The listing builds one solid part. Answer for the finished solid, in the listing's coordinates (mm). Face numbers are marked on the shaded views. A direction names the side the tool comes from. Give positions to 0.01 mm unless a question says otherwise; leave off trailing zeros. Write each loop counter-clockwise with the first axis right and the second up, starting at its lowest first coordinate (ties: lowest second). Pieces come first, ordered by that corner, then holes. Notation, with made-up numbers: M -28,20 L -12,20 A28 cw -12,56 Z; hole C -16,-35.75 d4. An arc over 180 degrees is marked long. Return JSON: item names as keys, results as strings.
Autodesk Inventor part; units mm, degrees
ref_plane "YZ Plane" through (0, 0, 0) normal (1, 0, 0) x (0, 1, 0)
ref_plane "XZ Plane" through (0, 0, 0) normal (0, 1, 0) x (-1, 0, 0)
ref_plane "XY Plane" through (0, 0, 0) normal (0, 0, 1) x (1, 0, 0)
sketch "Sketch1" plane through (0, 0, 0) normal (0, 0, 1) x (1, 0, 0)
  line L0 (0, 0) -> (34, 0)
  line L1 (34, 0) -> (34, 20)
  line L2 (34, 20) -> (0, 20)
  line L3 (0, 20) -> (0, 0)
  circle A0 centre (29, 10) radius 2.5
  point P0 (34, 10)
  dimension "d0" = 34
  dimension "d1" = 20
  dimension "d2" = 5
  dimension "d3" = 5
extrude "Extrusion1" add sketch "Sketch1" along normal blind 5
sketch "Sketch2" plane through (0, 0, 0) normal (-1, 0, 0) x (0, 0, 1)
  line L0 (0, 0) -> (0, 20)
  line L1 (0, 20) -> (34, 20)
  line L2 (34, 20) -> (34, 0)
  line L3 (34, 0) -> (0, 0)
  line L4 (0, 0) -> (0, 20)
  circle A0 centre (29, 10) radius 2.5
  point P0 (5, 0)
  point P1 (34, 10)
  dimension "d6" = 34
  dimension "d7" = 5
  dimension "d8" = 5
extrude "Extrusion2" add sketch "Sketch2" against normal blind 5
sketch "Sketch3" plane through (0, 20, 0) normal (0, 1, 0) x (1, 0, 0)
  line L0 (34, -5) -> (5, -5)
  line L1 (5, -5) -> (5, -34)
  line L2 (5, -34) -> (5, -5)
  line L3 (5, -34) -> (34, -5)
  point P0 (0, 0)
extrude "Extrusion3" add sketch "Sketch3" against normal blind 2
sketch "Sketch4" plane through (0, 0, 0) normal (0, -1, 0) x (1, 0, 0)
  line L0 (34, 5) -> (5, 5)
  line L1 (34, 5) -> (5, 34)
  line L2 (5, 5) -> (5, 34)
  point P0 (0, 0)
extrude "Extrusion4" add sketch "Sketch4" against normal blind 2
sketch "Sketch5" plane through (0, 18, 0) normal (0, -1, 0) x (1, 0, 0)
  line L0 (5, 31.5) -> (5, 26.5)
  line L1 (26.5, 5) -> (31.5, 5)
  line L2 (5, 26.5) -> (5, 5)
  line L3 (5, 5) -> (26.5, 5)
  line L4 (5, 21) -> (21, 5)
  line L5 (29, 5) -> (29, 0)
  line L6 (34, 0) -> (0, 0)
  line L7 (5, 29) -> (0, 29)
  line L8 (5, 21) -> (18, 21)
  line L9 (21, 5) -> (21, 18)
  line L10 (5, 34) -> (34, 5)
  line L11 (18, 21) -> (21, 18)
  dimension "d15" = 8
  dimension "d16" = 8
extrude "Extrusion5" add sketch "Sketch5" along normal blind 16
properties part number "L Bracket Small"
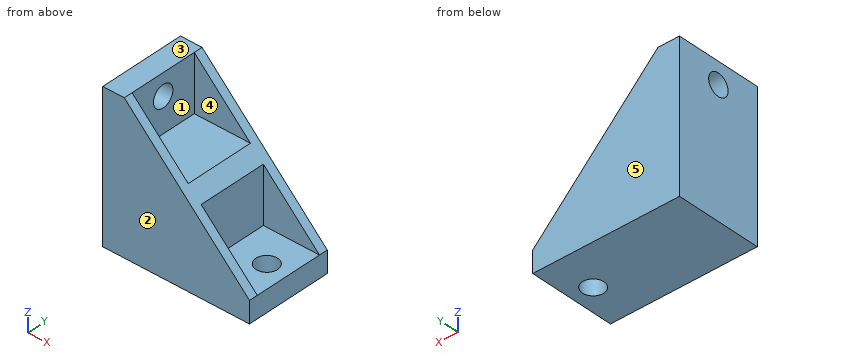
Item 1: A cutting plane is placed at D-D, the plane z = 22. Write down the section's boundary in (x, y).
Geometry results:
{"outline": "M 0,0 L 17,0 L 17,2 L 5,2 L 5,18 L 17,18 L 17,20 L 0,20 Z"}
Item 2: Which of the six approach directions +Z, -Z, +X, -X, +Y, -Y give full straight-line access (tool end or side, diameter ignored) to the marked faces 1 and 2?
Geometry results:
{"face 1": "+Z, +X", "face 2": "+Z, -Z, +X, -X, -Y"}
Item 3: A cutting plane is placed at C-C, the plane y = 10. Write down the section's boundary in (x, z).
Geometry results:
{"outline": "M 0,0 L 26.5,0 L 26.5,5 L 21,5 L 21,18 L 18,21 L 5,21 L 5,26.5 L 0,26.5 Z; M 0,31.5 L 5,31.5 L 5,34 L 0,34 Z; M 31.5,0 L 34,0 L 34,5 L 31.5,5 Z"}
Item 4: Find the intervals of material crossed by line 1 (Y direction, x = 26.5, z = 8); line 2 (Y direction, x = 3, z = 29); line 3 (Z direction, x = 14, y = 4.75), in increasing order.
Geometry results:
{"line 1": "y = 0 to 2, 18 to 20", "line 2": "y = 0 to 7.5, 12.5 to 20", "line 3": "z = 0 to 21"}
Item 5: Given pin 1 Ø10.5 at (x, z) = (14.5, 25) entering from +Y; pin 2 Ø8 at (x, y) = (17.5, 10.5) entering from +Z; pin 3 Ø4 at (y, z) = (3.5, 25.5) entering from +X; pin 4 Ø4.5 at (y, z) = (10, 29) entering from +X, each flat-ended and moving along its own axis, determine where each tip first touches the part or whether it passes through.
Geometry results:
{"pin 1": "stops at y = 20", "pin 2": "stops at z = 21", "pin 3": "stops at x = 14.82", "pin 4": "passes through"}
Item 6: Determine the mould class of the marked faces 3, 4 and 5 for opening direction Y: +Y half, -Y half, draft (parallel to the pull), parting line (faces both ways), or undercut.
Geometry results:
{"face 3": "draft", "face 4": "undercut", "face 5": "+Y half"}
Item 7: A cutting plane is placed at A-A, the plane z = 29. Write down the section's boundary in (x, y), plus the area to 3 significant figures.
Geometry results:
{"outline": "M 0,0 L 10,0 L 10,2 L 5,2 L 5,7.5 L 0,7.5 Z; M 0,12.5 L 5,12.5 L 5,18 L 10,18 L 10,20 L 0,20 Z", "area": "95.0 mm2"}
Item 8: A cutting plane is placed at B-B, the plane x = 29. Write down the section's boundary in (y, z).
Geometry results:
{"outline": "M 0,0 L 7.5,0 L 7.5,5 L 2,5 L 2,10 L 0,10 Z; M 12.5,0 L 20,0 L 20,10 L 18,10 L 18,5 L 12.5,5 Z"}
